Part print with two shaded views. Sizes in mm from the minimum x, y, z corner. Round coordinates to 2 decimals unless told otherwise and drop trailing zeros. Loops run counter-clockwise (first coordinate to the right, second up) from the corner with the lowest first, then second, coordinate; pieces in that order, holes last.
(1) Cut at D-D on y = 3.35. List the corners of the cut face in (x, z), then the cut area to 3 significant figures.
(2) Cut at B-B on z = 10. List the corners of the cut face in (x, y), then the cut area to 3 significant figures.
(3) Flat gauge pins, fed straight in: pin 1 (7.5 mm diameter, centred on x = 10, z = 110, fed in from +Y); pin 2 (1 mm diameter, centred on y = 3, z = 94, fed in from -X). Where does each tip first touch, or does it go through?
(4) Cut at A-A on z = 110. List the corners of the cut face in (x, y), then the cut area to 3 significant figures.
(5) Probe probe 1 along Z at (x, y) = (110, 3.1); probe 2 along Z at (x, y) = (57, 1); probe 3 along Z at (x, y) = (62.5, 3.6). List the from-to ranges inside material, lowest first.
(6) Cut at C-C on x = 60. List the corners of the cut face in (y, z), then the cut area to 3 significant figures.
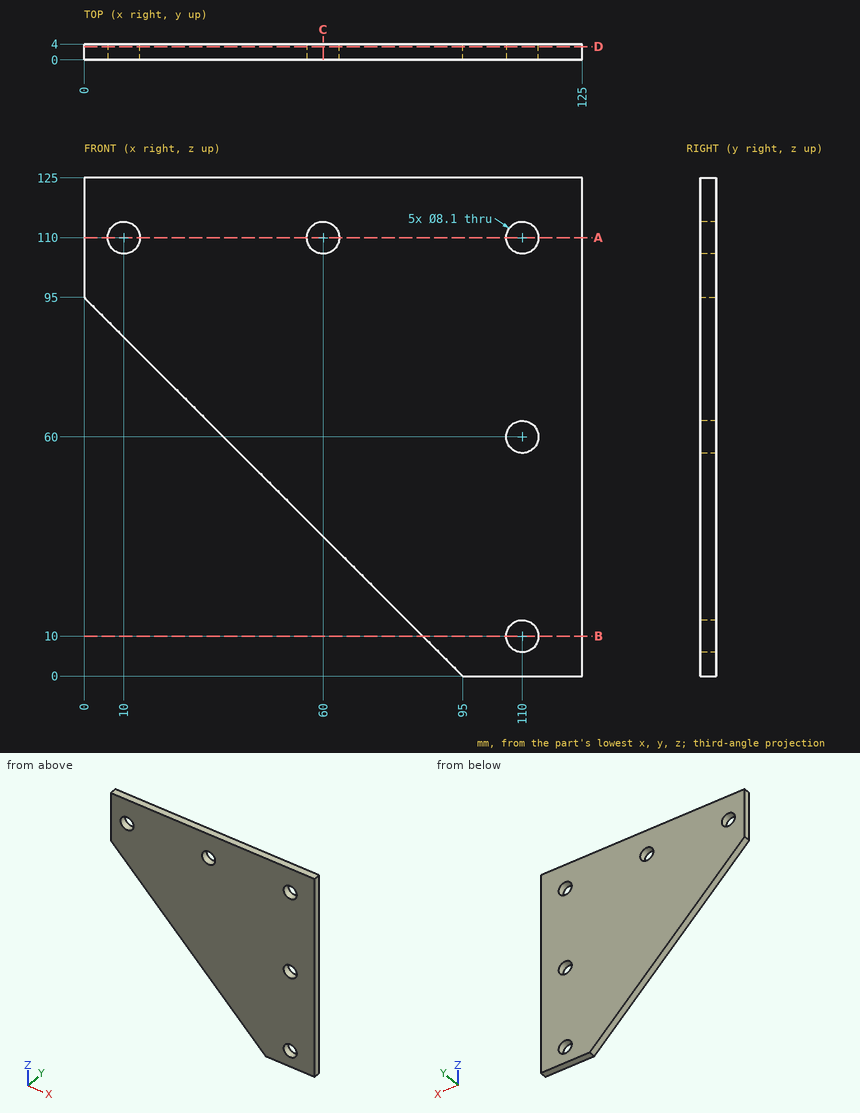
Final values:
1. outline: (0, 95) - (95, 0) - (125, 0) - (125, 125) - (0, 125) - close; hole circle Ø8.1 at (10, 110); hole circle Ø8.1 at (60, 110); hole circle Ø8.1 at (110, 10); hole circle Ø8.1 at (110, 60); hole circle Ø8.1 at (110, 110)
1. area: 10,900 mm2
2. outline: (85, 0) - (105.95, 0) - (105.95, 4) - (85, 4) - close; (114.05, 0) - (125, 0) - (125, 4) - (114.05, 4) - close
2. area: 128 mm2
3. pin 1: passes through
3. pin 2: stops at x = 0.5
4. outline: (0, 0) - (5.95, 0) - (5.95, 4) - (0, 4) - close; (14.05, 0) - (55.95, 0) - (55.95, 4) - (14.05, 4) - close; (64.05, 0) - (105.95, 0) - (105.95, 4) - (64.05, 4) - close; (114.05, 0) - (125, 0) - (125, 4) - (114.05, 4) - close
4. area: 403 mm2
5. probe 1: z = 0 to 5.95, 14.05 to 55.95, 64.05 to 105.95, 114.05 to 125
5. probe 2: z = 38 to 107.28, 112.72 to 125
5. probe 3: z = 32.5 to 106.81, 113.19 to 125
6. outline: (0, 35) - (4, 35) - (4, 105.95) - (0, 105.95) - close; (0, 114.05) - (4, 114.05) - (4, 125) - (0, 125) - close
6. area: 328 mm2
